from build123d import *

# Parameters (mm, degrees)
BOSS_EXTRUDE1_DEPTH     = 40
SKETCH3_W               = 90
SKETCH3_H               = 40
CUT_EXTRUDE_THIN1_DEPTH = 80
SKETCH4_R               = 15
BOSS_EXTRUDE2_DEPTH     = 80


with BuildPart() as part:
    # Sketch2 → Boss-Extrude1 (new, symmetric)
    with BuildSketch(Plane(origin=(0, 0, 0), x_dir=(1, 0, 0), z_dir=(0, 1, 0))):
        with BuildLine():
            Line((0, 40), (300, 40))
            ThreePointArc((300, 40), (340, 0), (300, -40))
            Line((300, -40), (0, -40))
            ThreePointArc((0, -40), (-40, 0), (0, 40))
        make_face()
    extrude(amount=BOSS_EXTRUDE1_DEPTH, both=True)

    # Sketch3 → Cut-Extrude-Thin1 (cut)
    with BuildSketch(Plane.XY.offset(40)):
        with Locations((5, 0)):
            Rectangle(SKETCH3_W, SKETCH3_H)
        with Locations((295, 0)):
            Rectangle(SKETCH3_W, SKETCH3_H)
    extrude(amount=-CUT_EXTRUDE_THIN1_DEPTH, mode=Mode.SUBTRACT)

    # Sketch4 → Boss-Extrude2 (add)
    with BuildSketch(Plane.XZ.offset(40)):
        Circle(SKETCH4_R)
        with Locations(Location((300, 0, 0), (0, 0, 180))):
            Circle(SKETCH4_R)
    extrude(amount=-BOSS_EXTRUDE2_DEPTH)


solid = part.part
Could you check a few things on this model? Use its own coordinates, in mm. A direction names the side the tool comes from. Give positions to 0.01 mm unless a question says otherwise; leave off trailing zeros. Order: outer loops, then holes, each group sorted by start corner. A loop starts at its lowest first (then second) coordinate and runs counter-clockwise, first axis right, second up. Notation, with made-up numbers: (-9.75, 14.25) -> (46.25, 14.25) arc R16 cw to (46.25, 38.25) -> close; hole circle Ø9 at (58, 38). An arc over 180 degrees is marked (long way). Answer in a Markdown table with one row per item. Add a question column.
Item 1: We'd pull the mould along X, two halves only. Please class faces 1 (the flat face through (147, -40, 1)), 2 (the cylindrical face through (-39.99, -29.86, 0.88)), 3 (the flat face through (250, 0, 1)): pulls with the +X half, pulls with the -X half, needs draft (parallel to the pull), parting line crosses it, or undercut.
Item 2: Imagine slicing it at D-D (y = 28). List the corners of the cut face in (x, z) for me, and give its area (3 significant figures).
Item 3: Please list where these lines run through material, in increasing order: probe 1 along X at (y, z) = (19, -4); probe 2 along Y at (x, z) = (41.5, 4.5); probe 3 along X at (y, z) = (-8, -3).
Item 4: Imagine slicing it at C-C (z = 28). List the corners of the cut face in (x, y) for me, and give its area (3 significant figures).
Item 5: Imagine slicing it at A-A (y = 0.5). List the corners of the cut face in (x, z) for me, and give its area (3 significant figures).
Item 6: I'm going to push flat-ended pins straight in: P1, Ø4, axis at y = -4, z = 15, coming from the -X side; P2, Ø1, axis at y = -3, z = -17, coming from the -X side; P3, Ø12, axis at y = -1, z = -10, coming from the -X side. Where does each tip first touch, or does it pass through?
Item 7: For faces 4 (the cylindrical face through (-14.985, -0.28, 0.66)), 5 (the flat face through (50, 0, 1)), 6 (the cylindrical face through (-39.99, 30.14, 0.88)), which set-ups out of +Z, -Z, +X, -X, +Y, -Y let a thin tool reach every point of the face, with its end or its side?
Item 8: Imagine slicing it at B-B (z = 0). List the corners of the cut face in (x, y) for me.
Result:
| question | item | result |
|---|---|---|
| 1 | face 1 | needs draft |
| 1 | face 2 | pulls with the -X half |
| 1 | face 3 | undercut |
| 2 | outline | (0, -40) -> (300, -40) arc R40 ccw to (300, 40) -> (0, 40) arc R40 ccw to start |
| 2 | area | 29,000 mm2 |
| 3 | probe 1 | -14.46 to 14.46, 50 to 250, 285.54 to 314.46 |
| 3 | probe 2 | -40 to -20, 20 to 40 |
| 3 | probe 3 | -14.7 to 14.7, 50 to 250, 285.3 to 314.7 |
| 4 | outline | (-28.57, -40) -> (328.57, -40) -> (328.57, -20) -> (250, -20) -> (250, 20) -> (328.57, 20) -> (328.57, 40) -> (-28.57, 40) -> (-28.57, 20) -> (50, 20) -> (50, -20) -> (-28.57, -20) -> close |
| 4 | area | 22,300 mm2 |
| 5 | outline | circle Ø30 at (0, 0); (50, -40) -> (250, -40) -> (250, 40) -> (50, 40) -> close; circle Ø30 at (300, 0) |
| 5 | area | 17,400 mm2 |
| 6 | P1 | x = -7.48 |
| 6 | P2 | x = 50 |
| 6 | P3 | x = -14.46 |
| 7 | face 4 | none |
| 7 | face 5 | +Z, -Z |
| 7 | face 6 | -X, +Y, -Y |
| 8 | outline | (-40, -40) -> (340, -40) -> (340, -20) -> (315, -20) -> (315, 20) -> (340, 20) -> (340, 40) -> (-40, 40) -> (-40, 20) -> (-15, 20) -> (-15, -20) -> (-40, -20) -> close; hole (15, -20) -> (50, -20) -> (50, 20) -> (15, 20) -> close; hole (250, -20) -> (285, -20) -> (285, 20) -> (250, 20) -> close |
